For this review, take the finished solid that the model builds, in its own axes (mm). A direction names the side the tool comes from. Round coordinates to 2 decimals unless told otherwise and drop trailing zeros. Write each loop counter-clockwise with the first axis right and the second up, starting at its lowest first coordinate (ties: lowest second). Pieces come first, ordered by that corner, then holes. Notation, with made-up numbers: (-8.5, 29.25) - (37.5, 29.25) arc R5 cw to (37.5, 37.25) - close; hole circle Ø7 at (55, 60). An arc over 180 degrees is marked (long way). Answer in a Markdown table with one row per item. Add a question column.
from build123d import *

# Parameters (mm, degrees)
SKETCH1_R           = 5
SKETCH1_R_2         = 1.5
BOSS_EXTRUDE1_DEPTH = 6
FILLET1_R           = 2
SKETCH2_W           = 111
SKETCH2_H           = 8
CUT_EXTRUDE1_DEPTH  = 4


with BuildPart() as part:
    # Sketch1 → Boss-Extrude1 (new body)
    with BuildSketch(Plane.XY):
        with BuildLine():
            Line((26.339134382, 7.5), (130, 7.5))
            ThreePointArc((130, 7.5), (137.5, 0), (130, -7.5))
            Line((130, -7.5), (26.339134382, -7.5))
            ThreePointArc((26.339134382, -7.5), (14.055289009, -8.081658399), (1.881366742, -9.821428571))
            ThreePointArc((1.881366742, -9.821428571), (-10, 0), (1.881366742, 9.821428571))
            ThreePointArc((1.881366742, 9.821428571), (14.055289009, 8.081658399), (26.339134382, 7.5))
        make_face()
        Circle(SKETCH1_R, mode=Mode.SUBTRACT)
        with Locations((130, 0)):
            Circle(SKETCH1_R_2, mode=Mode.SUBTRACT)
    extrude(amount=BOSS_EXTRUDE1_DEPTH)

    # Fillet1
    fillet1_edges = [part.edges().sort_by_distance(p)[0] for p in [
        (14.055289009, 8.081658399, 6),
        (-10, 0, 6),
        (14.055289009, -8.081658399, 6),
        (78.169567191, -7.5, 6),
        (137.5, 0, 6),
        (78.169567191, -7.5, 0),
        (14.055289009, -8.081658399, 0),
        (-10, 0, 0),
        (78.169567191, 7.5, 6),
        (14.055289009, 8.081658399, 0),
        (78.169567191, 7.5, 0),
        (137.5, 0, 0),
    ]]
    fillet(fillet1_edges, radius=FILLET1_R)

    # Sketch2 → Cut-Extrude1 (cut)
    with BuildSketch(Plane(origin=(0, 0, 0), x_dir=(-1, 0, 0), z_dir=(0, 0, -1))):
        with Locations((-67.5, 0)):
            Rectangle(SKETCH2_W, SKETCH2_H)
    extrude(amount=-CUT_EXTRUDE1_DEPTH, mode=Mode.SUBTRACT)


solid = part.part
Q1. Add section B-B on x = 102.5. State the section outline as (y, z) points, then the cut area to 3 significant figures.
Q2. Insertion check: pin 1 Ø2 at (y, z) = (-1, 1) entering from +X; pin 2 Ø1 at (x, z) = (69, 2.5) entering from +Y; pin 3 Ø3 at (x, z) = (80, 1.5) entering from -Y. Each pin has a flat end and moves straight along its axis. Give the tip position at first contact, or say it passes through.
Q3. To check wall thickness, follow probe 1 along Y at (x, z) = (130, 1.7); probe 2 along Y at (x, z) = (93.5, 2.05); probe 3 along X at (y, z) = (-2.25, 3.75). State the ranges of each line that lie inside material, in increasing order.
Q4. Add section A-A on y = 0. State the section outline as (x, z) points.
Q5. Draft analysis for pull direction Y (two halves, no side actions). For faces 1 (the face through (-10, 0, 3)), 2 (the face through (12, 0, 2)), 3 (the face through (65, 0, 6)), state which applies: released by +Y, released by -Y, zero draft, split by the parting line, or undercut.
Q6. Tool access review of faces 4 (the face through (68, 4, 2)), 5 (the face through (137.5, 0.16, 2.99)): name each direction out of +Z, -Z, +X, -X, +Y, -Y from which nothing blocks a thin tool from reaching the whole face with its end or side.
Answer sheet:
| question | item | result |
|---|---|---|
| 1 | outline | (-7.5, 2) arc R2 ccw to (-5.5, 0) - (-4, 0) - (-4, 4) - (4, 4) - (4, 0) - (5.5, 0) arc R2 ccw to (7.5, 2) - (7.5, 4) arc R2 ccw to (5.5, 6) - (-5.5, 6) arc R2 ccw to (-7.5, 4) - close |
| 1 | area | 54.6 mm² |
| 2 | pin 1 | stops at x = 137.48 |
| 2 | pin 2 | stops at y = 7.5 |
| 2 | pin 3 | stops at y = -7.5 |
| 3 | probe 1 | y = -7.48 to -1.5, 1.5 to 7.48 |
| 3 | probe 2 | y = -7.5 to -4, 4 to 7.5 |
| 3 | probe 3 | x = -9.74 to -4.47, 4.47 to 12, 123 to 137.15 |
| 4 | outline | (-10, 2) arc R2 ccw to (-8, 0) - (-5, 0) - (-5, 6) - (-8, 6) arc R2 ccw to (-10, 4) - close; (5, 0) - (12, 0) - (12, 4) - (123, 4) - (123, 0) - (128.5, 0) - (128.5, 6) - (5, 6) - close; (131.5, 0) - (135.5, 0) arc R2 ccw to (137.5, 2) - (137.5, 4) arc R2 ccw to (135.5, 6) - (131.5, 6) - close |
| 5 | face 1 | split by the parting line |
| 5 | face 2 | undercut |
| 5 | face 3 | zero draft |
| 6 | face 4 | -Z |
| 6 | face 5 | +Z, -Z, +X |
